Design review of the part built by this model. Coordinates are the model's own, in mm. Face numbers are marked on the shaded views. A direction names the side the tool comes from. Round coordinates to 2 decimals unless told otherwise and drop trailing zeros. Order: outer loops, then holes, each group sorted by start corner. A loop starts at its lowest first (then second) coordinate and runs counter-clockwise, first axis right, second up. Notation, with made-up numbers: (11.5, 56.5) - (21.5, 56.5) arc R18 ccw to (21.5, 67.5) - close; hole circle Ø1 at (9.25, 53). An arc over 180 degrees is marked (long way). Answer as a JSON object with one key per item and string values. Group by question number.
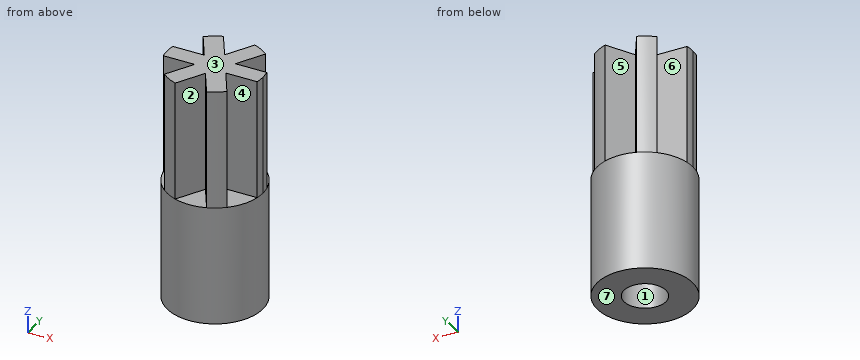
from build123d import *

# Parameters (mm, degrees)
F0_R     = 4
F0_R_2   = 1.75
F1_DEPTH = 10
F3_DEPTH = 8
F4_DEPTH = 10


with BuildPart() as f1:
    # F0 (on Top) → F1 (new body)
    with BuildSketch(Plane.XY):
        with Locations((-17.5178135131, 0)):
            Circle(F0_R)
        with Locations((-17.5178135131, 0)):
            Circle(F0_R_2, mode=Mode.SUBTRACT)
        with Locations((-17.5178135131, 0)):
            Circle(F0_R_2)
    extrude(amount=F1_DEPTH)

    # F0 (on Top) → F3 (cut)
    with BuildSketch(Plane.XY):
        with Locations((-17.5178135131, 0)):
            Circle(F0_R_2)
    extrude(amount=F3_DEPTH, mode=Mode.SUBTRACT)

    # F2 (on face) → F4 (join)
    with BuildSketch(Plane.XY.offset(10)):
        with BuildLine():
            Line((-16.6517881093, 0), (-13.5178135131, 0))
            ThreePointArc((-13.5178135131, 0), (-13.5355884036, 0.376673834), (-13.5887551017, 0.75))
            Line((-13.5887551017, 0.75), (-16.2187754074, 0.75))
            Line((-16.2187754074, 0.75), (-16.6517881093, 0))
        make_face()
        Polygon((-18.3838389169, 0), (-16.6517881093, 0), (-17.0848008112, 0.75), (-17.950826215, 0.75), align=None)
        with BuildLine():
            Line((-21.5178135131, 0), (-18.3838389169, 0))
            Line((-18.3838389169, 0), (-18.8168516188, 0.75))
            Line((-18.8168516188, 0.75), (-21.4468719245, 0.75))
            ThreePointArc((-21.4468719245, 0.75), (-21.5000386226, 0.376673834), (-21.5178135131, 0))
        make_face()
        with BuildLine():
            ThreePointArc((-13.5887551017, -0.75), (-13.5355884036, -0.376673834), (-13.5178135131, 0))
            Line((-13.5178135131, 0), (-16.6517881093, 0))
            Line((-16.6517881093, 0), (-16.2187754074, -0.75))
            Line((-16.2187754074, -0.75), (-13.5887551017, -0.75))
        make_face()
        Polygon((-17.0848008112, -0.75), (-16.6517881093, 0), (-18.3838389169, 0), (-17.950826215, -0.75), align=None)
        with BuildLine():
            Line((-18.8168516188, -0.75), (-18.3838389169, 0))
            Line((-18.3838389169, 0), (-21.5178135131, 0))
            ThreePointArc((-21.5178135131, 0), (-21.5000386226, -0.376673834), (-21.4468719245, -0.75))
            Line((-21.4468719245, -0.75), (-18.8168516188, -0.75))
        make_face()
        Polygon((-18.8168516188, 0.75), (-18.3838389169, 0), (-17.950826215, 0.75), align=None)
        Polygon((-17.0848008112, 0.75), (-16.6517881093, 0), (-16.2187754074, 0.75), align=None)
        Polygon((-16.2187754074, -0.75), (-16.6517881093, 0), (-17.0848008112, -0.75), align=None)
        Polygon((-17.950826215, -0.75), (-18.3838389169, 0), (-18.8168516188, -0.75), align=None)
        Polygon((-17.5178135131, -1.5), (-17.0848008112, -0.75), (-17.950826215, -0.75), align=None)
        with BuildLine():
            Line((-14.9037652546, -3.0276643972), (-16.2187754074, -0.75))
            Line((-16.2187754074, -0.75), (-17.0848008112, -0.75))
            Line((-17.0848008112, -0.75), (-17.5178135131, -1.5))
            Line((-17.5178135131, -1.5), (-16.2028033603, -3.7776643972))
            ThreePointArc((-16.2028033603, -3.7776643972), (-15.5178135131, -3.4641016151), (-14.9037652546, -3.0276643972))
        make_face()
        with BuildLine():
            Line((-17.5178135131, -1.5), (-17.950826215, -0.75))
            Line((-17.950826215, -0.75), (-18.8168516188, -0.75))
            Line((-18.8168516188, -0.75), (-20.1318617716, -3.0276643972))
            ThreePointArc((-20.1318617716, -3.0276643972), (-19.5178135131, -3.4641016151), (-18.832823666, -3.7776643972))
            Line((-18.832823666, -3.7776643972), (-17.5178135131, -1.5))
        make_face()
        Polygon((-17.950826215, 0.75), (-17.0848008112, 0.75), (-17.5178135131, 1.5), align=None)
        with BuildLine():
            Line((-20.1318617716, 3.0276643972), (-18.8168516188, 0.75))
            Line((-18.8168516188, 0.75), (-17.950826215, 0.75))
            Line((-17.950826215, 0.75), (-17.5178135131, 1.5))
            Line((-17.5178135131, 1.5), (-18.832823666, 3.7776643972))
            ThreePointArc((-18.832823666, 3.7776643972), (-19.5178135131, 3.4641016151), (-20.1318617716, 3.0276643972))
        make_face()
        with BuildLine():
            Line((-17.5178135131, 1.5), (-17.0848008112, 0.75))
            Line((-17.0848008112, 0.75), (-16.2187754074, 0.75))
            Line((-16.2187754074, 0.75), (-14.9037652546, 3.0276643972))
            ThreePointArc((-14.9037652546, 3.0276643972), (-15.5178135131, 3.4641016151), (-16.2028033603, 3.7776643972))
            Line((-16.2028033603, 3.7776643972), (-17.5178135131, 1.5))
        make_face()
    extrude(amount=F4_DEPTH)


solid = f1.part
1. Take a section at A-A, the plane z = 16.5. Give the boundary of the cut face in (x, y), then the cut area to 3 significant figures.
2. Tool access review of the marked faces 4, 5, 6 and 7: name each direction out of +Z, -Z, +X, -X, +Y, -Y from which nothing blocks a thin tool from reaching the whole face with its end or side.
3. Take a section at D-D, the plane z = 6. Give the boundary of the cut face in (x, y), then the cut area to 3 significant figures.
4. Take a section at C-C, the plane x = -18.5. Give the boundary of the cut face in (y, z), then the cut area to 3 significant figures.
5. Mouldability with a two-part tool opening along Y and no side actions: class the marked faces 1, 2 and 3 as pulls with the +Y half, pulls with the -Y half, needs draft (parallel to the pull), parting line crosses it, or undercut.
6. To check wall thickness, follow line 1 (Y direction, x = -15.5, z = 16.25); line 2 (Z direction, x = -16.25, y = -0.75); line 3 (Y direction, x = -18.5, z = 3.5). State the ranges of each line that lie inside material, in increasing order. Write a range as from..to.
7. Take a section at B-B, the plane y = -3.5. Give the boundary of the cut face in (x, z), then the cut area to 3 significant figures.
8. Clearance check with flat-ended pins moving along their axes: P1, Ø4.5, axis at x = -17.52, y = 0, coming from the -Z side; P2, Ø1, axis at x = -17.5, y = 0, coming from the -Z side; P3, Ø3, axis at x = -20.5, z = 16, coming from the +Y side; P4, Ø1.3, axis at x = -20, z = 17, coming from the -Y side. State where each tip first meets the part, or that it passes through.
Response values:
{
 "1": {"outline": "(-21.45, -0.75) - (-18.82, -0.75) - (-20.13, -3.03) arc R4 ccw to (-18.83, -3.78) - (-17.52, -1.5) - (-16.2, -3.78) arc R4 ccw to (-14.9, -3.03) - (-16.22, -0.75) - (-13.59, -0.75) arc R4 ccw to (-13.59, 0.75) - (-16.22, 0.75) - (-14.9, 3.03) arc R4 ccw to (-16.2, 3.78) - (-17.52, 1.5) - (-18.83, 3.78) arc R4 ccw to (-20.13, 3.03) - (-18.82, 0.75) - (-21.45, 0.75) arc R4 ccw to start", "area": "29.9 mm2"},
 "2": {"face 4": "+Z, +X", "face 5": "+Z, +Y", "face 6": "+Z, -X", "face 7": "-Z, +X, -X, +Y, -Y"},
 "3": {"outline": "circle Ø8 at (-17.52, 0); hole circle Ø3.5 at (-17.52, 0)", "area": "40.6 mm2"},
 "4": {"outline": "(-3.88, 0) - (-1.45, 0) - (-1.45, 8) - (1.45, 8) - (1.45, 0) - (3.88, 0) - (3.88, 10) - (3.2, 10) - (3.2, 20) - (-3.2, 20) - (-3.2, 10) - (-3.88, 10) - close", "area": "118 mm2"},
 "5": {"face 1": "undercut", "face 2": "pulls with the -Y half", "face 3": "needs draft"},
 "6": {"line 1": "-3.45..-1.99, -0.75..0.75, 1.99..3.45", "line 2": "8..20", "line 3": "-3.88..-1.45, 1.45..3.88"},
 "7": {"outline": "(-19.45, 0) - (-15.58, 0) - (-15.58, 20) - (-16.36, 20) - (-16.36, 10) - (-18.67, 10) - (-18.67, 20) - (-19.45, 20) - close", "area": "54.4 mm2"},
 "8": {"P1": "z = 0", "P2": "z = 8", "P3": "y = 3.72", "P4": "y = -3.56"}
}
